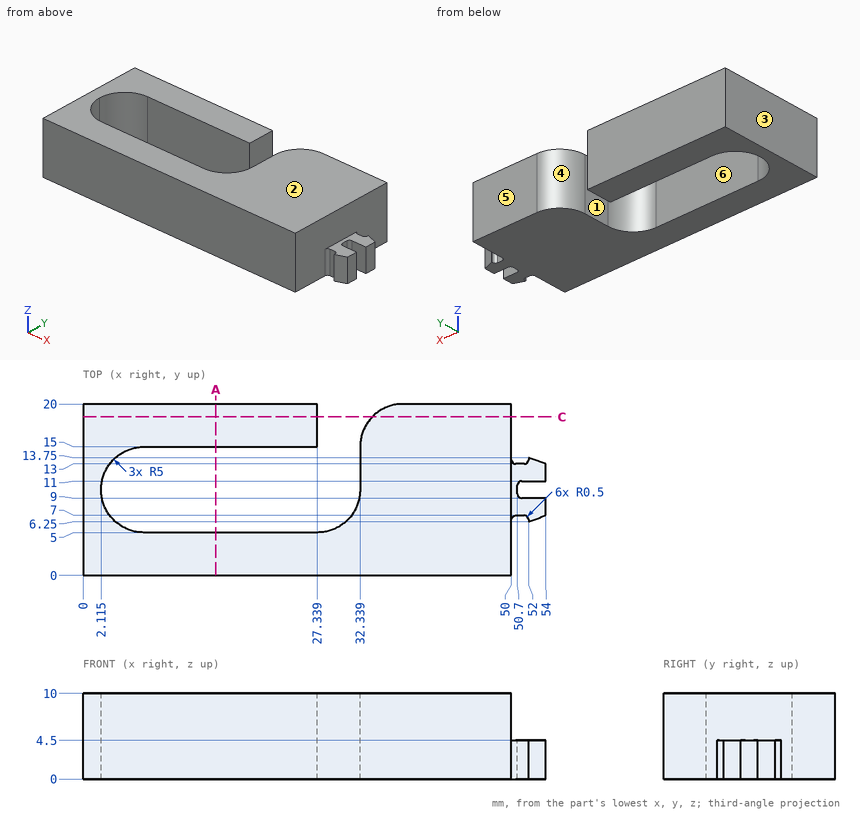
The figure shows three views and two pictorial views of one solid part (mm, origin at its lowest corner). Answer the questions. A direction names the side the tool comes from. Coordinates: 2 decimals unless noted, no trailing zeros. Write each loop counter-clockwise with the first axis right and the second up, starting at its lowest first coordinate (ties: lowest second). Pieces come first, ordered by that corner, then holes. Notation, with made-up numbers: (-3.5, 54.5) -> (32.5, 54.5) arc R26 ccw to (32.5, 90.5) -> close; hole circle Ø6 at (18.25, -24). An arc over 180 degrees is marked (long way). Return JSON: item names as keys, results as strings.
(1) The part is cut by section A-A on x = 15.5. Give the vertices of the cut face in (y, z).
Answers below:
{"outline": "(0, 0) -> (5, 0) -> (5, 10) -> (0, 10) -> close; (15, 0) -> (20, 0) -> (20, 10) -> (15, 10) -> close"}
(2) For a pull along X with two mould halves and no side action, classify the marked faces 1, 2 and 3 as pulls with the +X half, pulls with the -X half, needs draft (parallel to the pull), parting line crosses it, or undercut.
Answers below:
{"face 1": "undercut", "face 2": "needs draft", "face 3": "pulls with the -X half"}
(3) The part is cut by section C-C on y = 18.5. Give the vertices of the cut face in (x, z), then the cut area to 3 significant figures.
Answers below:
{"outline": "(0, 0) -> (27.34, 0) -> (27.34, 10) -> (0, 10) -> close; (33.77, 0) -> (50, 0) -> (50, 10) -> (33.77, 10) -> close", "area": "436 mm^2"}
(4) Which of the six approach directions +Z, -Z, +X, -X, +Y, -Y give full straight-line access (tool end or side, diameter ignored) to the marked faces 4, 5 and 6?
Answers below:
{"face 4": "+Z, -Z, +Y", "face 5": "+Z, -Z, +X, -X, +Y", "face 6": "+Z, -Z"}
(5) Each of these flat-tipped pins is pushed along its axis until it touches: P1, Ø1.2, axis at x = 51.5, y = 11.5, coming from the +Z side; P2, Ø0.5, axis at x = 51, z = 1.5, coming from the -Y side; P3, Ø0.8, axis at x = 51, z = 3, coming from the +Y side. Where does it stop, or does it pass through?
Answers below:
{"P1": "z = 4.5", "P2": "y = 7", "P3": "y = 13"}
(6) Consider line 1 along Y through (x, z) = (13, 2); line 2 along X through (y, z) = (9.75, 1.25); line 3 along X through (y, z) = (10, 8.5) (1 decimal). Determine where each line is inside the solid, lowest interval first. Write a range as from..to.
Answers below:
{"line 1": "0..5, 15..20", "line 2": "0..2.12, 32.33..50.7", "line 3": "0..2.1, 32.3..50"}
